Answer from the drawing. Dimensions are ordinates in mm from the lowest x, y and z of the part. Round coordinates to 2 decimals unless told otherwise and drop trailing zeros. Write each loop counter-clockwise with the first axis right and the second up, starting at its lowest first coordinate (ties: lowest second). Pieces come first, ordered by that corner, then holes.
1. Straight lines are drawn through the part: probe 1 along X at (y, z) = (18, 1.2); probe 2 along Y at (x, z) = (43, 0.3); probe 3 along X at (y, z) = (6, 0.45). For each, find the intervals that lie inside material, in ascending order.
2. Find section C-C (z = 1.45). Write down the section's boundary in (x, y), and give its area (3 significant figures).
3. Find section A-A (y = 14.5). Write down the section's boundary in (x, z).
4. Find section B-B (x = 56.5). Write down the section's boundary in (y, z).
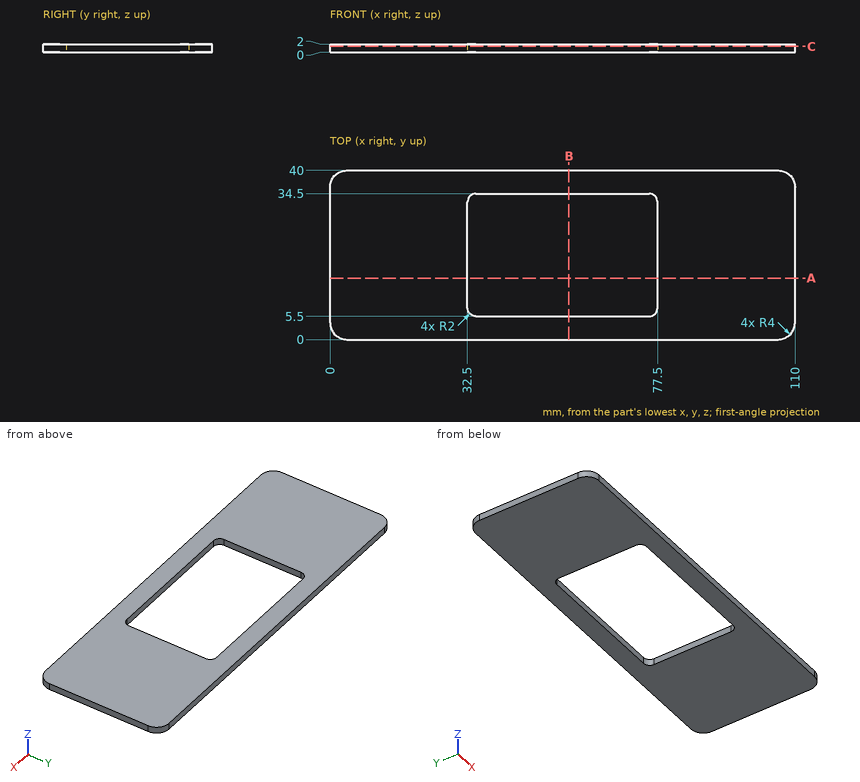
Worked answers:
1. probe 1: x = 0 to 32.5, 77.5 to 110
1. probe 2: y = 0 to 5.5, 34.5 to 40
1. probe 3: x = 0 to 33.18, 76.82 to 110
2. outline: (0, 4) arc R4 ccw to (4, 0) - (106, 0) arc R4 ccw to (110, 4) - (110, 36) arc R4 ccw to (106, 40) - (4, 40) arc R4 ccw to (0, 36) - close; hole (32.5, 7.5) arc R2 ccw to (34.5, 5.5) - (75.5, 5.5) arc R2 ccw to (77.5, 7.5) - (77.5, 32.5) arc R2 ccw to (75.5, 34.5) - (34.5, 34.5) arc R2 ccw to (32.5, 32.5) - close
2. area: 3,080 mm2
3. outline: (0, 0) - (32.5, 0) - (32.5, 2) - (0, 2) - close; (77.5, 0) - (110, 0) - (110, 2) - (77.5, 2) - close
4. outline: (0, 0) - (5.5, 0) - (5.5, 2) - (0, 2) - close; (34.5, 0) - (40, 0) - (40, 2) - (34.5, 2) - close
